Autodesk Inventor part; units mm, degrees
ref_plane "YZ Plane" through (0, 0, 0) normal (1, 0, 0) x (0, 1, 0)
ref_plane "XZ Plane" through (0, 0, 0) normal (0, 1, 0) x (-1, 0, 0)
ref_plane "XY Plane" through (0, 0, 0) normal (0, 0, 1) x (1, 0, 0)
sketch "Sketch1" plane through (0, 0, 0) normal (0, 1, 0) x (-1, 0, 0)
  circle A0 centre (0, 0) radius 425
  circle A1 centre (0, 0) radius 233.71
  dimension "d84" = 467.42
  dimension "d85" = 850
extrude "Extrusion3" add sketch "Sketch1" along normal blind 6
sketch "Sketch2" plane through (0, 6, 0) normal (0, 1, 0) x (1, 0, 0)
  circle A0 centre (0, 0) radius 329.355 construction
  line L0 (3.25, 363.0217) -> (3.25, 295.6883)
  line L1 (-3.25, 295.6883) -> (-3.25, 363.0217)
  arc A1 (-3.25, 295.6883) -> (-1.9167, 294.355) centre (-1.9167, 295.6883) ccw
  arc A2 (1.9167, 294.355) -> (3.25, 295.6883) centre (1.9167, 295.6883) ccw
  arc A3 (-1.9167, 364.355) -> (-3.25, 363.0217) centre (-1.9167, 363.0217) ccw
  arc A4 (3.25, 363.0217) -> (1.9167, 364.355) centre (1.9167, 363.0217) ccw
  line L2 (-1.9167, 364.355) -> (1.9167, 364.355)
  line L3 (-1.9167, 294.355) -> (1.9167, 294.355)
  line L4 (0, 294.355) -> (0, 329.355) construction
  line L5 (0, 364.355) -> (0, 329.355) construction
  line L6 (0, 364.355) -> (0, 294.355) construction
  line L7 (175.0629, -238.5433) -> (171.9617, -240.7965)
  arc A5 (176.9253, -238.8383) -> (175.0629, -238.5433) centre (175.8467, -239.622) ccw
  arc A6 (171.9617, -240.7965) -> (171.6667, -242.6589) centre (172.7454, -241.8752) ccw
  line L8 (173.0175, -238.1382) -> (193.59, -266.4538) construction
  line L9 (211.2443, -297.1327) -> (171.6667, -242.6589)
  line L10 (176.9253, -238.8383) -> (216.5029, -293.3121)
  line L11 (214.1625, -294.7694) -> (173.0175, -238.1382) construction
  line L12 (214.1625, -294.7694) -> (193.59, -266.4538) construction
  arc A7 (211.2443, -297.1327) -> (213.1067, -297.4277) centre (212.323, -296.349) ccw
  line L13 (216.2079, -295.1745) -> (213.1067, -297.4277)
  arc A8 (216.2079, -295.1745) -> (216.5029, -293.3121) centre (215.4242, -294.0958) ccw
  line L14 (280.1548, 92.2019) -> (281.3393, 88.5562)
  arc A9 (281.0108, 93.882) -> (280.1548, 92.2019) centre (281.4229, 92.614) ccw
  arc A10 (281.3393, 88.5562) -> (283.0194, 87.7002) centre (282.6074, 88.9682) ccw
  line L15 (279.9482, 90.9607) -> (313.2352, 101.7763) construction
  line L16 (347.0573, 108.5073) -> (283.0194, 87.7002)
  line L17 (281.0108, 93.882) -> (345.0486, 114.6892)
  line L18 (346.5222, 112.5919) -> (279.9482, 90.9607) construction
  line L19 (346.5222, 112.5919) -> (313.2352, 101.7763) construction
  arc A11 (347.0573, 108.5073) -> (347.9133, 110.1874) centre (346.6452, 109.7754) ccw
  line L20 (346.7287, 113.8331) -> (347.9133, 110.1874)
  arc A12 (346.7287, 113.8331) -> (345.0486, 114.6892) centre (345.4607, 113.4211) ccw
  dimension "d86" = 658.71
  dimension "d21" = 6.5
  dimension "d24" = 2.6667
  dimension "d25" = 2.6667
  dimension "d32" = 1.3333
  dimension "d33" = 1.3333
  dimension "d162" = 70
  dimension "d163" = 294.355
  dimension "d165" = 3.25
extrude "Extrusion4" cut sketch "Sketch2" against normal through all
sketch "Sketch3" plane through (0, 6, 0) normal (0, 1, 0) x (1, 0, 0)
  arc A0 (-131.3389, -404.1968) -> (131.3445, -404.195) centre (0, 0) ccw
  arc A1 (-77.7244, -128.3741) -> (77.7297, -128.3709) centre (0, 0) ccw
  line L0 (-122.1811, -173.696) -> (-161.3589, -227.6196)
  line L1 (-131.3389, -404.1968) -> (-77.7244, -128.3741)
  line L2 (0, 0) -> (0, -341.2918)
  line L3 (131.3445, -404.195) -> (77.7297, -128.3709)
  line L4 (210.5535, -295.3313) -> (171.3679, -241.3969)
  dimension "d52" = 25
  dimension "d87" = 150.07
  dimension "d88" = 425
  dimension "d89" = 25
  dimension "d90" = 11
  dimension "d91" = 11
sketch "Sketch5" plane through (0, 6, 0) normal (0, 1, 0) x (1, 0, 0)
  line L0 (3.25, 363.0217) -> (3.25, 295.6883)
  line L1 (5.5862, 281.6788) -> (-6.155, 278.5328)
  line L2 (-11.2263, 385.43) -> (10.5847, 377.0575)
  line L3 (6.5657, 233.6709) -> (8.9394, 278.9635)
  line L4 (14.2034, 379.4075) -> (16.5771, 424.7001)
  arc A0 (10.5847, 377.0575) -> (14.2034, 379.4075) centre (11.5404, 379.5471) ccw
  arc A1 (8.9394, 278.9635) -> (5.5862, 281.6788) centre (6.2763, 279.103) ccw
  arc A2 (-11.2263, 385.43) -> (-14.8449, 382.8009) centre (-12.1819, 382.9405) ccw
  line L5 (-3.25, 295.6883) -> (-3.25, 363.0217)
  line L6 (-14.8449, 382.8009) -> (-9.5081, 280.969)
  arc A3 (-9.5081, 280.969) -> (-6.155, 278.5328) centre (-6.8451, 281.1086) ccw
  line L7 (-1.9167, 294.355) -> (1.9167, 294.355)
  line L8 (1.9167, 364.355) -> (-1.9167, 364.355)
  line L9 (16.5771, 424.7001) -> (16.5774, 424.7058)
  line L10 (6.5657, 233.6709) -> (6.5621, 233.6028)
  circle A4 centre (0, 0) radius 425
  circle A5 centre (0, 0) radius 233.71
  line L11 (-356.4489, 130.7516) -> (-398.7912, 147.0053)
  arc A6 (-355.3322, 126.5839) -> (-356.4489, 130.7516) centre (-357.4046, 128.2621) ccw
  line L12 (-370.0348, 108.4276) -> (-355.3322, 126.5839)
  arc A7 (-370.0348, 108.4276) -> (-368.6526, 104.1736) centre (-367.9624, 106.7494) ccw
  line L13 (-368.6526, 104.1736) -> (-270.1556, 77.7814)
  arc A8 (-270.1556, 77.7814) -> (-266.8024, 80.2177) centre (-269.4654, 80.3572) ccw
  line L14 (-266.1663, 92.3563) -> (-266.8024, 80.2177)
  arc A9 (-262.5476, 94.7063) -> (-266.1663, 92.3563) centre (-263.5032, 92.2167) ccw
  line L15 (-220.2053, 78.4526) -> (-262.5476, 94.7063)
  line L16 (-220.2053, 78.4526) -> (-220.1417, 78.4282)
  line L17 (-398.7912, 147.0053) -> (-398.7965, 147.0073)
  line L18 (-142.66, -185.1845) -> (-142.6172, -185.1316)
  line L19 (-263.0436, -333.8458) -> (-263.0472, -333.8502)
  line L20 (132.0366, -192.9029) -> (131.9995, -192.8458)
  line L21 (236.2213, -353.3334) -> (236.2244, -353.3381)
  line L22 (365.2271, 103.7351) -> (409.0364, 115.4738)
  arc A10 (361.8739, 106.4505) -> (365.2271, 103.7351) centre (364.5369, 106.3109) ccw
  line L23 (363.0966, 129.7812) -> (361.8739, 106.4505)
  arc A11 (363.0966, 129.7812) -> (359.478, 132.4103) centre (360.4336, 129.9208) ccw
  line L24 (359.478, 132.4103) -> (264.2793, 95.867)
  arc A12 (264.2793, 95.867) -> (262.9985, 91.9251) centre (265.2349, 93.3774) ccw
  line L25 (269.6187, 81.7308) -> (262.9985, 91.9251)
  arc A13 (268.0724, 77.7026) -> (269.6187, 81.7308) centre (267.3822, 80.2784) ccw
  line L26 (224.2631, 65.9639) -> (268.0724, 77.7026)
  line L27 (224.2631, 65.9639) -> (224.1973, 65.9463)
  line L28 (409.0364, 115.4738) -> (409.0419, 115.4753)
  line L29 (0, -233.71) -> (0, -425)
  arc A14 (131.3445, -404.195) -> (-131.3389, -404.1968) centre (0, 0) ccw
  point P0 (-425, 0)
  point P1 (-425, 0)
  point P2 (-398.7693, 146.9969)
  point P3 (-220.1557, 78.4336)
  point P4 (16.5759, 424.6766)
  point P5 (6.5629, 233.6178)
  dimension "d63" = 2.6667
  dimension "d64" = 3
  dimension "d66" = 3
  dimension "d67" = 2.6667
  dimension "d68" = 2.6667
  dimension "d70" = 72
  dimension "d71" = 72
sketch "Sketch6" plane through (0, 6, 0) normal (0, 1, 0) x (1, 0, 0)
  line L0 (237.9351, -331.8846) -> (247.6433, -324.8312)
  line L1 (243.8227, -319.5725) -> (234.1145, -326.626)
  line L2 (210.5535, -295.3313) -> (171.3679, -241.3969)
  line L3 (215.5172, -293.3731) -> (212.416, -295.6263)
  arc A0 (244.7539, -319.72) -> (243.8227, -319.5725) centre (244.2145, -320.1119) ccw
  arc A1 (247.6433, -324.8312) -> (247.7908, -323.9) centre (247.2514, -324.2918) ccw
  arc A2 (237.0039, -331.7371) -> (237.9351, -331.8846) centre (237.5432, -331.3452) ccw
  arc A3 (234.1145, -326.626) -> (233.967, -327.5572) centre (234.5063, -327.1653) ccw
  line L4 (233.967, -327.5572) -> (237.0039, -331.7371)
  line L5 (247.7908, -323.9) -> (244.7539, -319.72)
  line L6 (171.3679, -241.3969) -> (210.5535, -295.3313)
  line L7 (190.9607, -268.3641) -> (196.2193, -264.5435)
  line L8 (215.8122, -291.5107) -> (176.6265, -237.5763)
  line L9 (145.065, -204.0599) -> (154.7732, -197.0065)
  line L10 (158.5938, -202.2651) -> (148.8856, -209.3185)
  arc A4 (158.5938, -202.2651) -> (158.7413, -201.3339) centre (158.202, -201.7257) ccw
  arc A5 (155.7044, -197.154) -> (154.7732, -197.0065) centre (155.1651, -197.5458) ccw
  arc A6 (145.065, -204.0599) -> (144.9175, -204.9911) centre (145.4569, -204.5992) ccw
  arc A7 (147.9544, -209.171) -> (148.8856, -209.3185) centre (148.4938, -208.7792) ccw
  line L11 (147.9544, -209.171) -> (144.9175, -204.9911)
  line L12 (155.7044, -197.154) -> (158.7413, -201.3339)
  point P0 (0, 0)
  dimension "d104" = 6.5
  dimension "d105" = 12
  dimension "d108" = 1.3333
  dimension "d109" = 1.3333
  dimension "d110" = 1.3333
  dimension "d111" = 1.3333
  dimension "d112" = 0
  dimension "d149" = 145
  dimension "d150" = 90
  dimension "d151" = 90
  dimension "d152" = 90
  dimension "d153" = 90
extrude "Extrusion7" cut sketch "Sketch6" against normal through all
pattern_circular "Circular Pattern2" count 2 over 72 about axis through (0, -10, 0) along (0, 1, 0) of "Extrusion7"
pattern_circular "Circular Pattern3" count 2 over 144 about axis through (0, -10, 0) along (0, 1, 0) of "Extrusion7"
mirror "Mirror3" about plane through (0, 0, 0) normal (1, 0, 0) of "Extrusion7"
extrude "Extrusion10" cut sketch "Sketch3" against normal blind 10
mirror "Mirror4" about plane through (0, 0, 0) normal (1, 0, 0) of "Extrusion4"
pattern_circular "Circular Pattern4" count 2 over 144 about axis through (0, -10, 0) along (0, -1, 0) of "Extrusion7"
extrude "Extrusion11" cut sketch "Sketch5" against normal through all contours L1 A3 L6 A2 L2 A0 L4 A4 L22 A10 L23 A11 L24 A12 L25 A13 L26 L27 A5 L10 L3 A1 | L27 L26 A13 L25 A12 L24 A11 L23 A10 L22 A4 L29 A5 | A5 L29 A4 L11 A6 L12 A7 L13 A8 L14 A9 L15 L16
equation "\"BendRadius\" = Thickness"
equation "\"BendReliefWidth\" = Thickness"
equation "\"BendReliefDepth\" = 0.5 * Thickness"
equation "\"CornerReliefSize\" = 4 * Thickness"
equation "\"MinimumRemnant\" = 2 * Thickness"
equation "\"TransitionRadius\" = BendRadius"
equation "\"JacobiRadiusSize\" = BendRadius"
equation "\"GapSize\" = Thickness"
properties part number "Ring C2" material "Wood (Maple)"
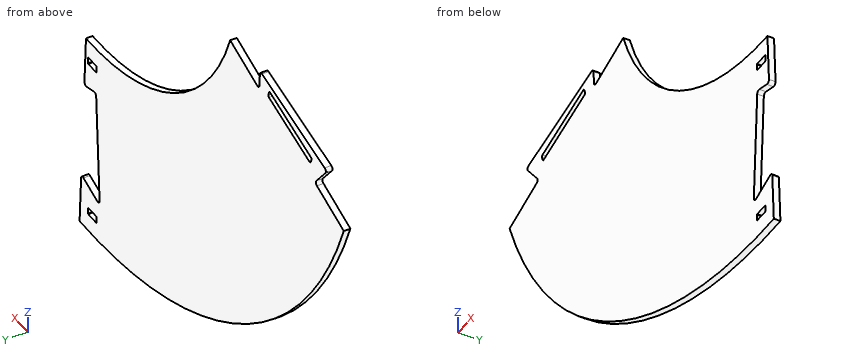
For this review, take the finished solid that the model builds, in its own axes (mm). Coordinates: 2 decimals unless noted, no trailing zeros. Loops run counter-clockwise (first coordinate to the right, second up) from the corner with the lowest first, then second, coordinate; pieces in that order, holes last. Notation, with made-up numbers: (23, 1.25) -> (31, 1.25) arc R20 ccw to (31, 12.25) -> close; hole circle Ø8 at (66, -36.5). An arc over 180 degrees is marked (long way). Return JSON: item names as keys, results as strings. Group by question number.
(1) Consider section C-C, the plane z = -159. Give the boundary of the cut face in (x, y), plus the area to 3 significant figures.
(2) Consider section D-D, the plane x = -83. Give the boundary of the cut face in (y, z), plus the area to 3 significant figures.
(3) Consider section A-A, the plane x = -291. Give the boundary of the cut face in (y, z).
(4) To check wall thickness, follow L1, parallel to Z at x = -304.5, y = 5.4; L2, parallel to X at y = 2.75, z = -253; L3, parallel to Z at x = -344, y = 1.4. State the ranges of each line that lie inside material, in increasing order.
(5) Consider section B-B, the plane y = 2.9. Count the separate pieces of the cut face and the enclosed holes in it, plus the area to 3 significant figures.
(6) For pin 1 Ø1.6 at (y, z) = (3, -405) entering from +X; pin 2 Ø1.5 at (x, y) = (-120, 3) entering from -Z; pin 3 Ø3 at (y, z) = (4.5, -112.5) entering from -X, all flat-tipped, find the tip position at first contact; note any pin that passes through.
Results below:
{
 "1": {"outline": "(-394.14, 0) -> (-171.29, 0) -> (-171.29, 6) -> (-394.14, 6) -> close", "area": "1,340 mm2"},
 "2": {"outline": "(0, -416.82) -> (6, -416.82) -> (6, -218.48) -> (0, -218.48) -> close", "area": "1,190 mm2"},
 "3": {"outline": "(0, -309.75) -> (6, -309.75) -> (6, -97.13) -> (0, -97.13) -> close; (0, -90.29) -> (6, -90.29) -> (6, -83.37) -> (0, -83.37) -> close"},
 "4": {"L1": "z = -296.49 to -101.51, -94.68 to -86.98", "L2": "x = -341.49 to -10.08, 3.25 to 7.58", "L3": "z = -249.58 to -114.35, -107.51 to -97.57"},
 "5": {"separate pieces": "1", "enclosed holes": "3", "area": "78,500 mm2"},
 "6": {"pin 1": "stops at x = 15.59", "pin 2": "stops at z = -407.93", "pin 3": "stops at x = -367.95"}
}
